from build123d import *

# Parameters (mm, degrees)
BOSS_EXTRUDE1_DEPTH = 4.953
SKETCH4_W           = 52.07
SKETCH4_H           = 19.05
SKETCH4_R           = 9.528566475
BOSS_EXTRUDE4_DEPTH = 4.953
SKETCH5_R           = 2.794
CUT_EXTRUDE1_DEPTH  = 4.953


with BuildPart() as part:
    # Sketch1 → Boss-Extrude1 (new body)
    with BuildSketch(Plane.XY):
        with BuildLine():
            Line((-41.509205492, 38.23442277), (-41.509205492, -12.56557723))
            Line((-41.509205492, -12.56557723), (-20.563828914, -12.56557723))
            ThreePointArc((-20.563828914, -12.56557723), (-14.071874854, -2.900775285), (-11.791205492, 8.51642277))
            ThreePointArc((-11.791205492, 8.51642277), (-20.495406169, 29.530222094), (-41.509205492, 38.23442277))
        make_face()
        with BuildLine():
            Line((-62.45458207, -12.56557723), (-41.509205492, -12.56557723))
            Line((-41.509205492, -12.56557723), (-41.509205492, 38.23442277))
            ThreePointArc((-41.509205492, 38.23442277), (-62.523004816, 29.530222094), (-71.227205492, 8.51642277))
            ThreePointArc((-71.227205492, 8.51642277), (-68.946536131, -2.900775285), (-62.45458207, -12.56557723))
        make_face()
        with BuildLine():
            ThreePointArc((-11.791205492, 8.51642277), (-14.071874854, -2.900775285), (-20.563828914, -12.56557723))
            Line((-20.563828914, -12.56557723), (9.711739651, -12.56557723))
            Line((9.711739651, -12.56557723), (295.040794508, -12.56557723))
            Line((295.040794508, -12.56557723), (295.040794508, 38.23442277))
            Line((295.040794508, 38.23442277), (-41.509205492, 38.23442277))
            ThreePointArc((-41.509205492, 38.23442277), (-20.495406169, 29.530222094), (-11.791205492, 8.51642277))
        make_face()
        with BuildLine():
            Line((-71.227205492, -12.56557723), (-62.45458207, -12.56557723))
            ThreePointArc((-62.45458207, -12.56557723), (-68.946536131, -2.900775285), (-71.227205492, 8.51642277))
            Line((-71.227205492, 8.51642277), (-71.227205492, -12.56557723))
        make_face()
    extrude(amount=BOSS_EXTRUDE1_DEPTH)

    # Sketch4 → Boss-Extrude4 (add)
    with BuildSketch(Plane(origin=(0, 0, 0), x_dir=(-1, 0, 0), z_dir=(0, 0, -1))):
        with Locations((171.684205492, -23.36057723)):
            Rectangle(SKETCH4_W, SKETCH4_H)
        with BuildLine():
            Line((145.649205492, -13.83557723), (93.579205492, -13.83557723))
            ThreePointArc((93.579205492, -13.83557723), (77.773954719, -7.288828003), (71.227205492, 8.51642277))
            Line((71.227205492, 8.51642277), (71.227205492, -12.56557723))
            Line((71.227205492, -12.56557723), (48.370059515, -12.56557723))
            ThreePointArc((48.370059515, -12.56557723), (56.179798103, -14.24000578), (62.61663913, -18.968938574))
            ThreePointArc((62.61663913, -18.968938574), (76.606040295, -29.246485846), (93.579205492, -32.88557723))
            Line((93.579205492, -32.88557723), (145.649205492, -32.88557723))
            Line((145.649205492, -32.88557723), (145.649205492, -13.83557723))
        make_face()
        with BuildLine():
            ThreePointArc((206.26970661, 31.017935339), (220.549824511, 5.053937718), (197.719205492, -13.83557723))
            Line((197.719205492, -13.83557723), (197.719205492, -32.88557723))
            ThreePointArc((197.719205492, -32.88557723), (239.658720339, 3.959196789), (208.522432887, 50.294840539))
            Line((208.522432887, 50.294840539), (207.444047034, 41.066936521))
            Line((207.444047034, 41.066936521), (206.26970661, 31.017935339))
        make_face()
        with Locations((197.979885508, 42.172931859)):
            Circle(SKETCH4_R)
        with BuildLine():
            Line((207.444047034, 41.066936521), (208.522432887, 50.294840539))
            ThreePointArc((208.522432887, 50.294840539), (203.499658151, 51.301032243), (198.392077595, 51.69257874))
            ThreePointArc((198.392077595, 51.69257874), (204.861788543, 48.763302841), (207.508451983, 42.172931859))
            ThreePointArc((207.508451983, 42.172931859), (207.492337119, 41.618997367), (207.444047034, 41.066936521))
        make_face()
        with BuildLine():
            ThreePointArc((198.088987461, 32.644990012), (202.252933463, 32.201450179), (206.26970661, 31.017935339))
            Line((206.26970661, 31.017935339), (207.444047034, 41.066936521))
            ThreePointArc((207.444047034, 41.066936521), (204.355161122, 35.091304933), (198.088987461, 32.644990012))
        make_face()
    extrude(amount=-BOSS_EXTRUDE4_DEPTH)

    # Sketch5 → Cut-Extrude1 (cut)
    with BuildSketch(Plane(origin=(0, 0, 0), x_dir=(-1, 0, 0), z_dir=(0, 0, -1))):
        with Locations((-279.419794508, 12.83442277)):
            Circle(SKETCH5_R)
        with Locations((-259.734794508, 12.83442277)):
            Circle(SKETCH5_R)
        with Locations((-233.064794508, 12.83442277)):
            Circle(SKETCH5_R)
        with Locations((-208.172794508, 12.83442277)):
            Circle(SKETCH5_R)
        with Locations((-172.612794508, 12.83442277)):
            Circle(SKETCH5_R)
        with Locations((-152.927794508, 12.83442277)):
            Circle(SKETCH5_R)
        with Locations((-121.177794508, 12.83442277)):
            Circle(SKETCH5_R)
        with Locations((-95.777794508, 12.83442277)):
            Circle(SKETCH5_R)
    extrude(amount=-CUT_EXTRUDE1_DEPTH, mode=Mode.SUBTRACT)


solid = part.part
For this review, take the finished solid that the model builds, in its own axes (mm). A direction names the side the tool comes from. Give positions to 0.01 mm unless a question says otherwise; leave off trailing zeros. Write each loop counter-clockwise with the first axis right and the second up, starting at its lowest first coordinate (ties: lowest second). Pieces come first, ordered by that corner, then holes. Notation, with made-up numbers: (-17.5, 77) -> (37.5, 77) arc R7 cw to (37.5, 85) -> close; hole circle Ø9 at (-31, 33.25). An arc over 180 degrees is marked (long way). Use CSV: the item, a comma, the result in double quotes.
Q1. Tool access review of faces 5 (the face through (91, 10, 0)), 6 (the face through (-77.949, -7.462, 2.442)): name each direction out of +Z, -Z, +X, -X, +Y, -Y from which nothing blocks a thin tool from reaching the whole face with its end or side.
Conclusion:
face 5,"-Z, +X, -X, +Y, -Y"
face 6,"+Z, -Z, +Y"
Q2. Mouldability with a two-part tool opening along Y and no side actions: class faces 1 (the face through (91, 10, 4.953)), 2 (the face through (-62.29, 29.76, 2.44)), 3 (the face through (-188.46, 42.54, 2.44)), 4 (the face through (-76.383, -29.145, 2.442)) as pulls with the +Y half, pulls with the -Y half, needs draft (parallel to the pull), parting line crosses it, or undercut.
Conclusion:
face 1,"needs draft"
face 2,"pulls with the +Y half"
face 3,"undercut"
face 4,"pulls with the -Y half"
Q3. Take a section at B-B, the plane z = 1.9. State how many separate pieces and enclosed holes the cut face has, then the cut area to 3 significant figures.
Conclusion:
separate pieces,"1"
enclosed holes,"8"
area,"22,900 mm2"
Q4. Take a section at A-A, the plane y = -6.5. Write out the cut boundary in (x, z).
Conclusion:
outline,"(-236.91, 0) -> (-214.67, 0) -> (-214.67, 4.95) -> (-236.91, 4.95) -> close; (-77.02, 0) -> (295.04, 0) -> (295.04, 4.95) -> (-77.02, 4.95) -> close"
Q5. For P1, Ø1.5, axis at x = -148.5, z = 3, coming from the +Y side; P2, Ø2, axis at x = 237.5, z = 3.5, coming from the -Y side; P3, Ø2.5, axis at x = 185, z = 2.5, coming from the +Y side, all flat-tipped, find the tip position at first contact; note any pin that passes through.
Conclusion:
P1,"y = -13.84"
P2,"y = -12.57"
P3,"y = 38.23"
Q6. Take a section at D-D, the plane y = -27. Write out the cut boundary in (x, z), then the cut area to 3 significant figures.
Conclusion:
outline,"(-219.24, 0) -> (-72.3, 0) -> (-72.3, 4.95) -> (-219.24, 4.95) -> close"
area,"728 mm2"
Q7. To check wall thickness, follow probe 1 along Y at (x, z) = (164, 1.95); probe 2 along X at (y, z) = (-5.5, 0.8); probe 3 along X at (y, z) = (28, 1.65). State the ranges of each line that lie inside material, in increasing order. Write a range as [from, to].
Conclusion:
probe 1,"[-12.57, 38.23]"
probe 2,"[-237.3, -215.55], [-76.17, 295.04]"
probe 3,"[-235.7, -211.66], [-63.95, 295.04]"
Q8. Take a section at C-C, the plane x = 26.5. Write out the cut boundary in (y, z), then the cut area to 3 significant figures.
Conclusion:
outline,"(-12.57, 0) -> (38.23, 0) -> (38.23, 4.95) -> (-12.57, 4.95) -> close"
area,"252 mm2"
